Design review of the part built by this model. Coordinates are the model's own, in mm. A direction names the side the tool comes from. Coordinates: 2 decimals unless noted, no trailing zeros. Loops run counter-clockwise (first coordinate to the right, second up) from the corner with the lowest first, then second, coordinate; pieces in that order, holes last. Notation, with made-up numbers: (-38.5, 46) -> (10.5, 46) arc R26 ccw to (10.5, 83) -> close; hole circle Ø4 at (51.25, -13.5). An arc over 180 degrees is marked (long way). One line per item, written item: value. Start each with the question number.
1. Draft analysis for pull direction Z (two halves, no side actions). For faces 1 (the flat face through (-3.9, -0.1, -3.5)), 2 (the flat face through (2, 2, 2.5)), 3 (the cylindrical face through (-0.072, -0.444, -1.455)), state which applies: pulls with the +Z half, pulls with the -Z half, needs draft (parallel to the pull), parting line crosses it, or undercut.
2. Machinability: for faces 4 (the flat face through (4.1, 0.2, -11.5)), 5 (the flat face through (0, 0.2, -13)), 6 (the flat face through (0, 0, -6)), 7 (the flat face through (-3.2, 3.5, 0)), which of the approach directions +Z, -Z, +X, -X, +Y, -Y give a long, thin tool a straight path to every point of the face, cutting with its end or side? Answer none if there is none.
3. Add section A-A on y = 3. Write out the cut boundary in (x, z) (3 decimals), plus the area to 3 significant figures.
4. Insertion check: pin 1 (3 mm diameter, centred on y = 3.5, z = -3.5, fed in from -X); pin 2 (0.5 mm diameter, centred on x = 4.5, z = -11.5, fed in from +Y); pin 3 (0.5 mm diameter, centred on x = -3.5, z = -3.5, fed in from -Y). Each pin has a flat end and moves straight along its axis. Give the tip position at first contact, or say it passes through.
5. Add section B-B on z = -2. Write out the cut boundary in (x, y).
6. For probe 1 along Y at (x, z) = (0, -4.75); probe 2 along Z at (x, y) = (-0.75, 5.25); probe 3 along Z at (x, y) = (-3.25, 4.5), list the stretches that pass through material, from the lowest coordinate up.
```python
from build123d import *

# Parameters (mm, degrees)
ESQUISSE1_R             = 3
BOSS_EXTRU_1_DEPTH      = 2.5
ESQUISSE2_W             = 7
ESQUISSE2_H             = 6
BOSS_EXTRU_2_DEPTH      = 12
ESQUISSE4_R             = 1.8
ENL_V_MAT_EXTRU_2_DEPTH = 15.5
CHANFREIN2_SIZE         = 0.125
ESQUISSE5_R             = 0.55
BOSS_EXTRU_3_DEPTH      = 1
CONG_1_R                = 0.1
BOSS_EXTRU_4_START      = -0.2
ESQUISSE6_W             = 1.7
ESQUISSE6_H             = 1
BOSS_EXTRU_4_DEPTH      = 0.3
ESQUISSE7_W             = 1
ESQUISSE7_H             = 1.7
BOSS_EXTRU_5_DEPTH      = 0.1
BOSS_EXTRU_5_DEPTH_BACK = 0.2


with BuildPart() as part:
    # Esquisse1 → Boss.-Extru.1 (new body)
    with BuildSketch(Plane.XY):
        with Locations((0, 3)):
            Circle(ESQUISSE1_R)
    extrude(amount=BOSS_EXTRU_1_DEPTH)

    # Esquisse2 → Boss.-Extru.2 (add)
    with BuildSketch(Plane.XY):
        with Locations((0, 3)):
            Rectangle(ESQUISSE2_W, ESQUISSE2_H)
    extrude(amount=-BOSS_EXTRU_2_DEPTH)

    # Esquisse4 → Enlèv. mat.-Extru.2 (cut, through all)
    with BuildSketch(Plane.XY.offset(2.5)):
        with Locations((0, 3)):
            Circle(ESQUISSE4_R)
    extrude(amount=-ENL_V_MAT_EXTRU_2_DEPTH, mode=Mode.SUBTRACT)

    # Chanfrein2
    chanfrein2_edges = [part.edges().sort_by_distance(p)[0] for p in [
        (-1.8, 3, 2.5),
        (-3, 3, 2.5),
    ]]
    chamfer(chanfrein2_edges, length=CHANFREIN2_SIZE)

    # Esquisse5 → Boss.-Extru.3 (add)
    with BuildSketch(Plane.XZ):
        with Locations((0, -2)):
            Circle(ESQUISSE5_R)
        with Locations((0, -9)):
            Circle(ESQUISSE5_R)
    extrude(amount=BOSS_EXTRU_3_DEPTH)

    # Congé1
    cong_1_edges = [part.edges().sort_by_distance(p)[0] for p in [
        (-0.55, -1, -2),
        (-0.55, -1, -9),
    ]]
    fillet(cong_1_edges, radius=CONG_1_R)

    # Esquisse6 → Boss.-Extru.4 (add)
    with BuildSketch(Plane.XZ.offset(BOSS_EXTRU_4_START)):
        with Locations((-3.85, -3.5)):
            Rectangle(ESQUISSE6_W, ESQUISSE6_H)
        with Locations((-3.85, -11.5)):
            Rectangle(ESQUISSE6_W, ESQUISSE6_H)
    boss_extru_4 = extrude(amount=BOSS_EXTRU_4_DEPTH)

    # Symétrie1: Boss.-Extru.4 across plane
    add(boss_extru_4.mirror(Plane(origin=(0, 0, 0), x_dir=(0, 0, 1), z_dir=(1, 0, 0))))

    # Esquisse7 → Boss.-Extru.5 (add, two sides)
    with BuildSketch(Plane.XZ) as boss_extru_5_sk:
        with Locations((0, -12.35)):
            Rectangle(ESQUISSE7_W, ESQUISSE7_H)
    extrude(amount=BOSS_EXTRU_5_DEPTH)
    extrude(boss_extru_5_sk.sketch, amount=-BOSS_EXTRU_5_DEPTH_BACK)


solid = part.part
```
Worked answers:
1. face 1: needs draft
1. face 2: pulls with the +Z half
1. face 3: undercut
2. face 4: +Z, -Z, +X, +Y
2. face 5: -Z, +X, -X, +Y
2. face 6: -Y
2. face 7: +Z, -X
3. outline: (-3.5, -12) -> (-1.8, -12) -> (-1.8, 2.375) -> (-1.925, 2.5) -> (-2.875, 2.5) -> (-3, 2.375) -> (-3, 0) -> (-3.5, 0) -> close; (1.8, -12) -> (3.5, -12) -> (3.5, 0) -> (3, 0) -> (3, 2.375) -> (2.875, 2.5) -> (1.925, 2.5) -> (1.8, 2.375) -> close
3. area: 46.8 mm²
4. pin 1: stops at x = -3.5
4. pin 2: stops at y = 0.2
4. pin 3: stops at y = -0.1
5. outline: (-3.5, 0) -> (-0.55, 0) -> (-0.55, -0.9) arc R0.1 ccw to (-0.45, -1) -> (0.45, -1) arc R0.1 ccw to (0.55, -0.9) -> (0.55, 0) -> (3.5, 0) -> (3.5, 6) -> (-3.5, 6) -> close; hole circle Ø3.6 at (0, 3)
6. probe 1: y = 0 to 1.2, 4.8 to 6
6. probe 2: z = -12 to 2.5
6. probe 3: z = -12 to 0
